from build123d import *

# Parameters (mm, degrees)
SKETCH_1_R          = 35.8
EXTRUDE_1_DEPTH     = 47.7
SKETCH_2_R          = 5.25
EXTRUDE_2_DEPTH     = 20
SKETCH_3_W          = 7.138794325
SKETCH_3_H          = 6.164414002
CUT_EXTRUDE_1_DEPTH = 11
SKETCH_4_R          = 1.5
CUT_EXTRUDE_2_DEPTH = 87.422985947
CHAMFER_1_SIZE      = 1
SKETCH_5_R          = 1.65
CUT_EXTRUDE_3_DEPTH = 6
SKETCH_6_R          = 2.1
CUT_EXTRUDE_4_DEPTH = 24
SKETCH_7_R          = 30
EXTRUDE_3_DEPTH     = 15.8
SKETCH_8_W          = 3.2
SKETCH_8_H          = 12
CUT_EXTRUDE_5_DEPTH = 68.4


with BuildPart() as part:
    # 草图1 → 凸台-拉伸1 (new body)
    with BuildSketch(Plane(origin=(0, 0, 0), x_dir=(1, 0, 0), z_dir=(0, 1, 0))):
        with Locations(Location((0, 0, 0), (0, 0, 270))):
            Circle(SKETCH_1_R)
    extrude(amount=EXTRUDE_1_DEPTH)

    # 草图2 → 凸台-拉伸2 (add)
    with BuildSketch(Plane(origin=(0, 47.7, 0), x_dir=(1, 0, 0), z_dir=(0, 1, 0))):
        with Locations(Location((0, 0, 0), (0, 0, 270))):
            Circle(SKETCH_2_R)
    extrude(amount=EXTRUDE_2_DEPTH)

    # 草图3 → 切除-拉伸1 (cut)
    with BuildSketch(Plane(origin=(0, 67.7, 0), x_dir=(1, 0, 0), z_dir=(0, 1, 0))):
        with Locations((7.819397163, 0)):
            Rectangle(SKETCH_3_W, SKETCH_3_H)
    extrude(amount=-CUT_EXTRUDE_1_DEPTH, mode=Mode.SUBTRACT)

    # 草图4 → 切除-拉伸2 (cut, through all)
    with BuildSketch(Plane(origin=(4.25, 0, 0), x_dir=(0, 0, -1), z_dir=(1, 0, 0))):
        with Locations((0, 64.7)):
            Circle(SKETCH_4_R)
    extrude(amount=-CUT_EXTRUDE_2_DEPTH, mode=Mode.SUBTRACT)

    # 倒角1
    chamfer_1_edges = [part.edges().sort_by_distance(p)[0] for p in [
        (0, 47.7, -5.25),
    ]]
    chamfer(chamfer_1_edges, length=CHAMFER_1_SIZE)

    # 草图5 → 切除-拉伸3 (cut)
    with BuildSketch(Plane(origin=(0, 47.7, 0), x_dir=(1, 0, 0), z_dir=(0, 1, 0))):
        with Locations(Location((0, -20, 0), (0, 0, 270))):
            Circle(SKETCH_5_R)
        with Locations(Location((-17.320508076, 10, 0), (0, 0, 270))):
            Circle(SKETCH_5_R)
        with Locations(Location((17.320508076, 10, 0), (0, 0, 270))):
            Circle(SKETCH_5_R)
    extrude(amount=-CUT_EXTRUDE_3_DEPTH, mode=Mode.SUBTRACT)

    # 草图6 → 切除-拉伸4 (cut)
    with BuildSketch(Plane(origin=(0, 67.7, 0), x_dir=(1, 0, 0), z_dir=(0, 1, 0))):
        with Locations(Location((0, 0, 0), (0, 0, 270))):
            Circle(SKETCH_6_R)
    extrude(amount=-CUT_EXTRUDE_4_DEPTH, mode=Mode.SUBTRACT)

    # 草图7 → 凸台-拉伸3 (add)
    with BuildSketch(Plane.XZ):
        with Locations(Location((0, 0, 0), (0, 0, 90))):
            Circle(SKETCH_7_R)
    extrude(amount=EXTRUDE_3_DEPTH)

    # 草图8 → 切除-拉伸5 (cut, symmetric)
    with BuildSketch(Plane(origin=(0, 0, 0), x_dir=(0, 0, -1), z_dir=(1, 0, 0))):
        with Locations((28.4, -6)):
            Rectangle(SKETCH_8_W, SKETCH_8_H)
    extrude(amount=CUT_EXTRUDE_5_DEPTH, both=True, mode=Mode.SUBTRACT)


solid = part.part
Geometry: final body of the model. Coordinates: model frame, mm. A direction names the side the tool comes from. Give positions to 0.01 mm unless a question says otherwise; leave off trailing zeros. Loops run counter-clockwise (first coordinate to the right, second up) from the corner with the lowest first, then second, coordinate; pieces in that order, holes last. Notation, with made-up numbers: M 8.5,-26.5 L 33.5,-26.5 A25 ccw 33.5,8.5 Z; hole C 12.5,-21 d11. An arc over 180 degrees is marked long. Put each result on its own line as item: value.
1) Reachability of faces 5 (the cylindrical face through (11.49, -7.789, 27.712)), 6 (the cylindrical face through (15.71, 44.74, -10.36)), 7 (the flat face through (0, -6, -26.8)), 8 (the flat face through (4.25, 62, 0)) from +Z, -Z, +X, -X, +Y, -Y: full face, straight path, thin tool, end or side. Return the list, or none.
Computed values:
face 5: -Y
face 6: +Y
face 7: -Z, +X, -X
face 8: +Z, -Z, +X, +Y
2) Material intervals for L1, parallel to X at y = 57.75, z = 0; L2, parallel to Y at x = -3.9, z = 0; L3, parallel to X at y = 45, z = -10 (1 decimal), sorted ascending. Write a range as from..to.
Computed values:
L1: x = -5.25..-2.1, 2.1..4.25
L2: y = -15.8..63.2, 66.2..67.7
L3: x = -34.4..-19, -15.7..15.7, 19..34.4
3) First-contact query: P1, Ø1, axis at x = -18, z = -9.5, coming from the +Y side; P2, Ø0.8, axis at x = 4.5, z = -0.5, coming from the +Y side; P3, Ø5, axis at x = 18.5, z = -22.5, coming from the +Y side; P4, Ø7, axis at y = 62, z = -1, coming from the +X side. Flat tips, straight axial feed; report the tip coordinate or a pass-through.
Computed values:
P1: stops at y = 41.7
P2: stops at y = 67.7
P3: stops at y = 47.7
P4: stops at x = 4.25
4) Cut plane B-B, the plane y = 45.5. Return the cut outline in (x, z).
Computed values:
outline: C 0,0 d71.6; hole C -17.32,-10 d3.3; hole C 0,0 d4.2; hole C 0,20 d3.3; hole C 17.32,-10 d3.3
5) Cut plane A-A, the plane y = 64.7. Return the cut outline in (x, z).
Computed values:
outline: M -5.03,-1.5 A5.25 ccw 4.25,-3.08 L 4.25,-1.5 L 1.47,-1.5 A2.1 cw -1.47,-1.5 Z; M -5.03,1.5 L -1.47,1.5 A2.1 cw 1.47,1.5 L 4.25,1.5 L 4.25,3.08 A5.25 ccw Z
6) Mould query, pull axis Y, two halves, no side actions, for faces 1 (the cylindrical face through (-1, 44.74, 18.69)), 2 (the flat face through (0, -12, -28)), 3 (the cylindrical face through (2.879, 65.965, -0.806)), 4 (the flat face through (0, 43.7, 0)). Classes: released by +Y, released by -Y, zero draft, split by the parting line, or undercut.
Computed values:
face 1: zero draft
face 2: undercut
face 3: undercut
face 4: released by +Y
7) Cut plane D-D, the plane z = -10. Return the cut outline in (x, y) (1 decimal), plus the area to 3 significant figures.
Computed values:
outline: M -34.4,0 L -28.3,0 L -28.3,-15.8 L 28.3,-15.8 L 28.3,0 L 34.4,0 L 34.4,47.7 L 19,47.7 L 19,41.7 L 15.7,41.7 L 15.7,47.7 L -15.7,47.7 L -15.7,41.7 L -19,41.7 L -19,47.7 L -34.4,47.7 Z
area: 4,130 mm^2
8) Cut plane C-C, the plane x = 12. Return the cut outline in (y, z), plus the area to 3 significant figures.
Computed values:
outline: M -15.8,-27.5 L -12,-27.5 L -12,-26.8 L 0,-26.8 L 0,-33.73 L 47.7,-33.73 L 47.7,33.73 L 0,33.73 L 0,27.5 L -15.8,27.5 Z
area: 4,080 mm^2
